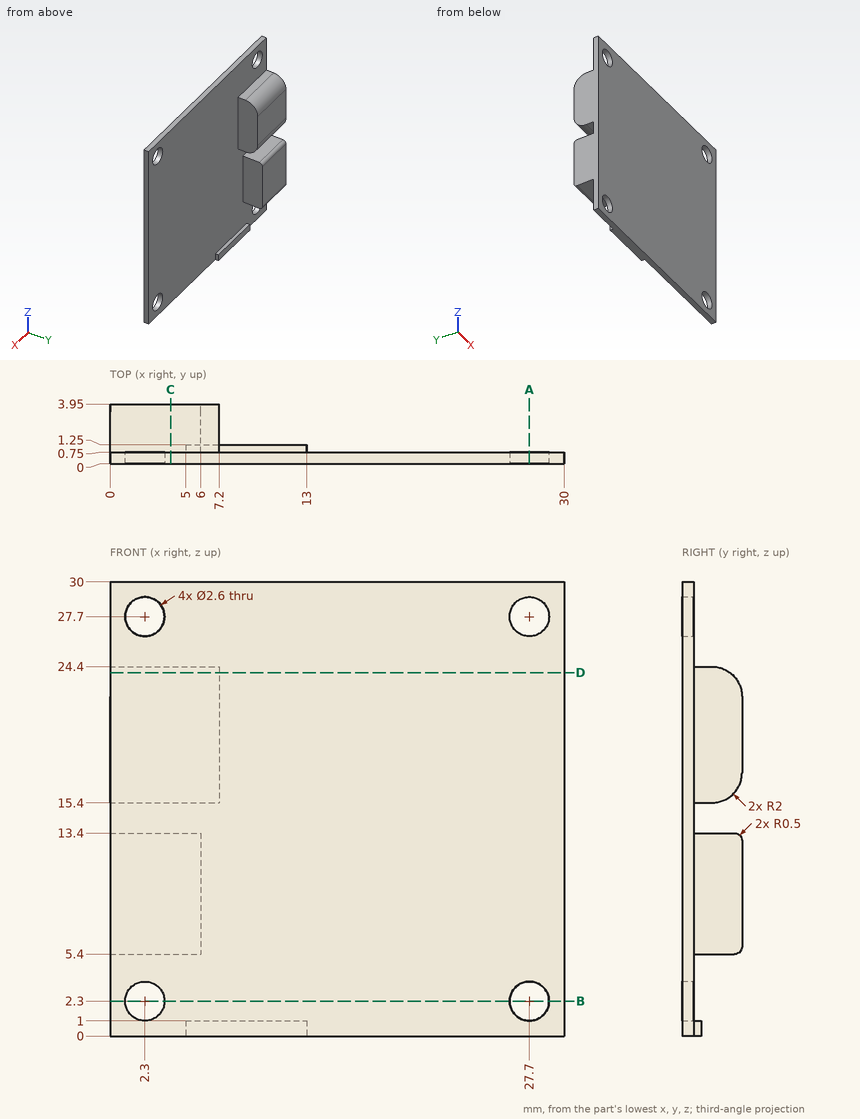
Input: dimensioned drawing with shaded views. Units: mm. Origin: part minimum x, y, z. Give positions to 0.01 mm unless a question says otherwise; leave off trailing zeros. Write each loop counter-clockwise with the first axis right and the second up, starting at its lowest first coordinate (ties: lowest second). Pieces come first, ordered by that corner, then holes.
1. First-contact query: pin 1 (2.5 mm diameter, centred on x = 27.7, z = 2.3, fed in from +Y); pin 2 (1 mm diameter, centred on y = 3, z = 10.5, fed in from +X); pin 3 (2 mm diameter, centred on x = 24.5, z = 5.5, fed in from +Y); pin 4 (1.3 mm diameter, centred on x = 3, y = 1.5, fed in from -Z). Flat tips, straight axial feed; report the tip coordinate or a pass-through.
2. Section query B-B (z = 2.3). Return the cut outline in (x, y).
3. Material intervals for line 1 along Z through (x, y) = (27.7, 0.4); line 2 along Z through (x, y) = (2.25, 2.05); line 3 along Y through (x, z) = (24.5, 22.5), sorted ascending.
4. Section query D-D (z = 24). Return the cut outline in (x, y), then the cut area to 3 significant figures.
5. Section query C-C (x = 4). Return the cut outline in (y, z), then the cut area to 3 significant figures.
6. Section query A-A (x = 27.7). Return the cut outline in (y, z), then the cut area to 3 significant figures.
Output values:
1. pin 1: passes through
1. pin 2: stops at x = 6
1. pin 3: stops at y = 0.75
1. pin 4: stops at z = 5.4
2. outline: (0, 0) - (1, 0) - (1, 0.75) - (0, 0.75) - close; (3.6, 0) - (26.4, 0) - (26.4, 0.75) - (3.6, 0.75) - close; (29, 0) - (30, 0) - (30, 0.75) - (29, 0.75) - close
3. line 1: z = 0 to 1, 3.6 to 26.4, 29 to 30
3. line 2: z = 5.4 to 13.4, 15.4 to 24.4
3. line 3: y = 0 to 0.75
4. outline: (0, 0) - (30, 0) - (30, 0.75) - (7.2, 0.75) - (7.2, 3.15) - (0, 3.15) - close
4. area: 39.8 mm2
5. outline: (0, 0) - (0.75, 0) - (0.75, 5.4) - (3.45, 5.4) arc R0.5 ccw to (3.95, 5.9) - (3.95, 12.9) arc R0.5 ccw to (3.45, 13.4) - (0.75, 13.4) - (0.75, 15.4) - (1.95, 15.4) arc R2 ccw to (3.95, 17.4) - (3.95, 22.4) arc R2 ccw to (1.95, 24.4) - (0.75, 24.4) - (0.75, 30) - (0, 30) - close
5. area: 75.1 mm2
6. outline: (0, 0) - (0.75, 0) - (0.75, 1) - (0, 1) - close; (0, 3.6) - (0.75, 3.6) - (0.75, 26.4) - (0, 26.4) - close; (0, 29) - (0.75, 29) - (0.75, 30) - (0, 30) - close
6. area: 18.6 mm2
